from build123d import *

# Parameters (mm, degrees)
SKETCH1_W            = 31.75
SKETCH1_H            = 15.875
BOSS_EXTRUDE1_DEPTH  = 1.4097
SKETCH2_W            = 29.21
SKETCH2_H            = 13.335
SKETCH2_R            = 3.175
SKETCH2_R_2          = 2.413
CUT_EXTRUDE1_DEPTH   = 1.5494
SKETCH3_R            = 2.69875
BOSS_EXTRUDE2_DEPTH  = 1.397
LPATTERN1_COUNT      = 4
LPATTERN1_PITCH      = 7.9375
LPATTERN1_COUNT_DIR2 = 2
LPATTERN1_PITCH_DIR2 = 7.9375
SKETCH2_3_R          = 3.175
SKETCH2_3_R_2        = 2.413
BOSS_EXTRUDE3_DEPTH  = 1.5494
LPATTERN2_COUNT      = 2
LPATTERN2_PITCH      = 7.9375
LPATTERN2_COL_COUNT  = 2
LPATTERN2_COL_PITCH  = 7.9375


with BuildPart() as part:
    # Sketch1 → Boss-Extrude1 (new, symmetric)
    with BuildSketch(Plane(origin=(0, 0, 0), x_dir=(1, 0, 0), z_dir=(0, 1, 0))):
        Rectangle(SKETCH1_W, SKETCH1_H)
    extrude(amount=BOSS_EXTRUDE1_DEPTH, both=True)

    # Sketch2 → Cut-Extrude1 (cut)
    with BuildSketch(Plane.XZ.offset(1.4097)):
        Rectangle(SKETCH2_W, SKETCH2_H)
        Circle(SKETCH2_R, mode=Mode.SUBTRACT)
        Circle(SKETCH2_R)
        Circle(SKETCH2_R_2, mode=Mode.SUBTRACT)
        Circle(SKETCH2_R_2)
    extrude(amount=-CUT_EXTRUDE1_DEPTH, mode=Mode.SUBTRACT)

    # Sketch3 → Boss-Extrude2 (add)
    with BuildSketch(Plane(origin=(0, 1.4097, 0), x_dir=(1, 0, 0), z_dir=(0, 1, 0))):
        with Locations(Location((11.90625, -3.96875, 0), (0, 0, 90))):
            Circle(SKETCH3_R)
    boss_extrude2 = extrude(amount=BOSS_EXTRUDE2_DEPTH)

    # LPattern1: Boss-Extrude2 4 × 2
    with Locations(*[(-i * LPATTERN1_PITCH, 0, -j * LPATTERN1_PITCH_DIR2) for i in range(LPATTERN1_COUNT) for j in range(LPATTERN1_COUNT_DIR2) if (i, j) != (0, 0)]):
        add(boss_extrude2)

    # Sketch2<3> → Boss-Extrude3 (add)
    with BuildSketch(Plane.XZ.offset(1.4097)):
        with Locations(Location((0, 0, 0), (0, 0, 270))):
            Circle(SKETCH2_3_R)
        with Locations(Location((0, 0, 0), (0, 0, 270))):
            Circle(SKETCH2_3_R_2, mode=Mode.SUBTRACT)
    boss_extrude3 = extrude(amount=-BOSS_EXTRUDE3_DEPTH)

    # LPattern2: Boss-Extrude3 ×2
    with Locations(*[(i * LPATTERN2_PITCH, 0, 0) for i in range(1, LPATTERN2_COUNT)]):
        add(boss_extrude3)

    # LPattern2 col: Boss-Extrude3 ×2
    with Locations(*[(-i * LPATTERN2_COL_PITCH, 0, 0) for i in range(1, LPATTERN2_COL_COUNT)]):
        add(boss_extrude3)


solid = part.part
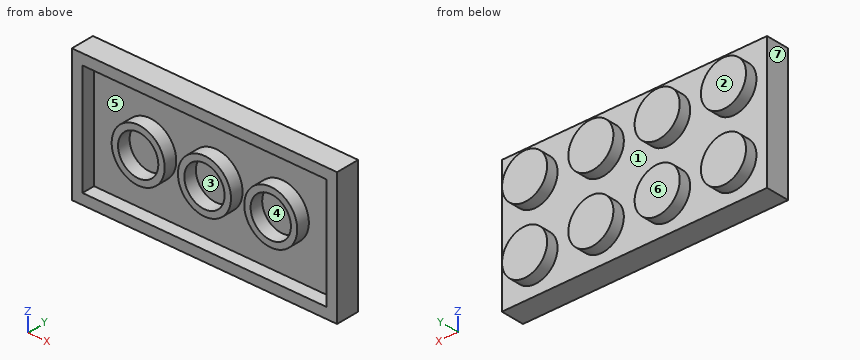
Build history of the part. All positions in model axes, mm. Face numbers are marked on the shaded views. A direction names the side the tool comes from. Coordinates: 2 decimals unless noted, no trailing zeros. Order: outer loops, then holes, each group sorted by start corner. A loop starts at its lowest first (then second) coordinate and runs counter-clockwise, first axis right, second up. Notation, with made-up numbers: (-39.5, 81) -> (-1.5, 81) arc R24 cw to (-1.5, 103) -> close; hole circle Ø7 at (82.25, 25.5). An arc over 180 degrees is marked (long way). One line per item, written item: value.
(1) Probe line 1 (X direction, y = -0.8, z = -6.5) (3 decimals); line 2 (Z direction, x = -12, y = 1.85); line 3 (Y direction, x = 11, z = 4.5). List the from-to ranges inside material, lowest first. Write a range as [from, to].
Checked values:
line 1: [-15.875, -14.605], [14.605, 15.875]
line 2: [-6.67, -1.27], [1.27, 6.67]
line 3: [0.14, 2.81]
(2) Drop flat-ended pins along their axis: pin 1 Ø2 at (x, z) = (-0.5, 0.5) entering from +Y; pin 2 Ø1.4 at (x, z) = (-8, -1) entering from -Y. Give the stop position or say it passes through.
Checked values:
pin 1: y = 1.41
pin 2: y = 0.14
(3) Slice it at D-D, the plane x = 12.5. List the corners of the cut face in (y, z).
Checked values:
outline: (-1.41, -7.94) -> (1.41, -7.94) -> (1.41, -6.6) -> (2.81, -6.6) -> (2.81, -1.34) -> (1.41, -1.34) -> (1.41, 1.34) -> (2.81, 1.34) -> (2.81, 6.6) -> (1.41, 6.6) -> (1.41, 7.94) -> (-1.41, 7.94) -> (-1.41, 6.67) -> (0.14, 6.67) -> (0.14, -6.67) -> (-1.41, -6.67) -> close
(4) Tool access for the marked faces 1, 2 and 3: list every direction of +Z, -Z, +X, -X, +Y, -Y with a clear straight run to the whole face (end or side of a thin tool).
Checked values:
face 1: +Y
face 2: +Z, -Z, +X, -X, +Y
face 3: -Y
(5) Slice it at B-B, the plane x = 0. List the corners of the cut face in (y, z) (1 decimal), plus the area to 3 significant figures.
Checked values:
outline: (-1.4, -7.9) -> (1.4, -7.9) -> (1.4, 7.9) -> (-1.4, 7.9) -> (-1.4, 6.7) -> (0.1, 6.7) -> (0.1, 3.2) -> (-1.4, 3.2) -> (-1.4, 2.4) -> (0.1, 2.4) -> (0.1, -2.4) -> (-1.4, -2.4) -> (-1.4, -3.2) -> (0.1, -3.2) -> (0.1, -6.7) -> (-1.4, -6.7) -> close
area: 26.5 mm2
(6) Slice it at C-C, the plane y = 2.05. List the corners of the cut face in (x, z), plus the area to 3 significant figures.
Checked values:
outline: circle Ø5.4 at (-11.91, -3.97); circle Ø5.4 at (-11.91, 3.97); circle Ø5.4 at (-3.97, -3.97); circle Ø5.4 at (-3.97, 3.97); circle Ø5.4 at (3.97, -3.97); circle Ø5.4 at (3.97, 3.97); circle Ø5.4 at (11.91, -3.97); circle Ø5.4 at (11.91, 3.97)
area: 183 mm2
(7) Mould opens along X. For the marked faces 4, 5, 6 and 7 say: pulls with the +X half, pulls with the -X half, needs draft (parallel to the pull), parting line crosses it, or undercut.
Checked values:
face 4: undercut
face 5: undercut
face 6: needs draft
face 7: pulls with the -X half
